Could you check a few things on this drawing? It's one solid part, dimensions in mm from its lowest x, y, z. A direction names the side the tool comes from. Give positions to 0.01 mm unless a question says otherwise; leave off trailing zeros. Write each loop counter-clockwise with the first axis right and the second up, starting at its lowest first coordinate (ties: lowest second). Pieces come first, ordered by that corner, then holes. Notation, with made-up numbers: M -40,45 L -8,45 A22 ccw -8,65 Z; hole C 47.25,8 d2. An arc over 180 degrees is marked long. Answer as CSV lines item,"result". Start each with the question number.
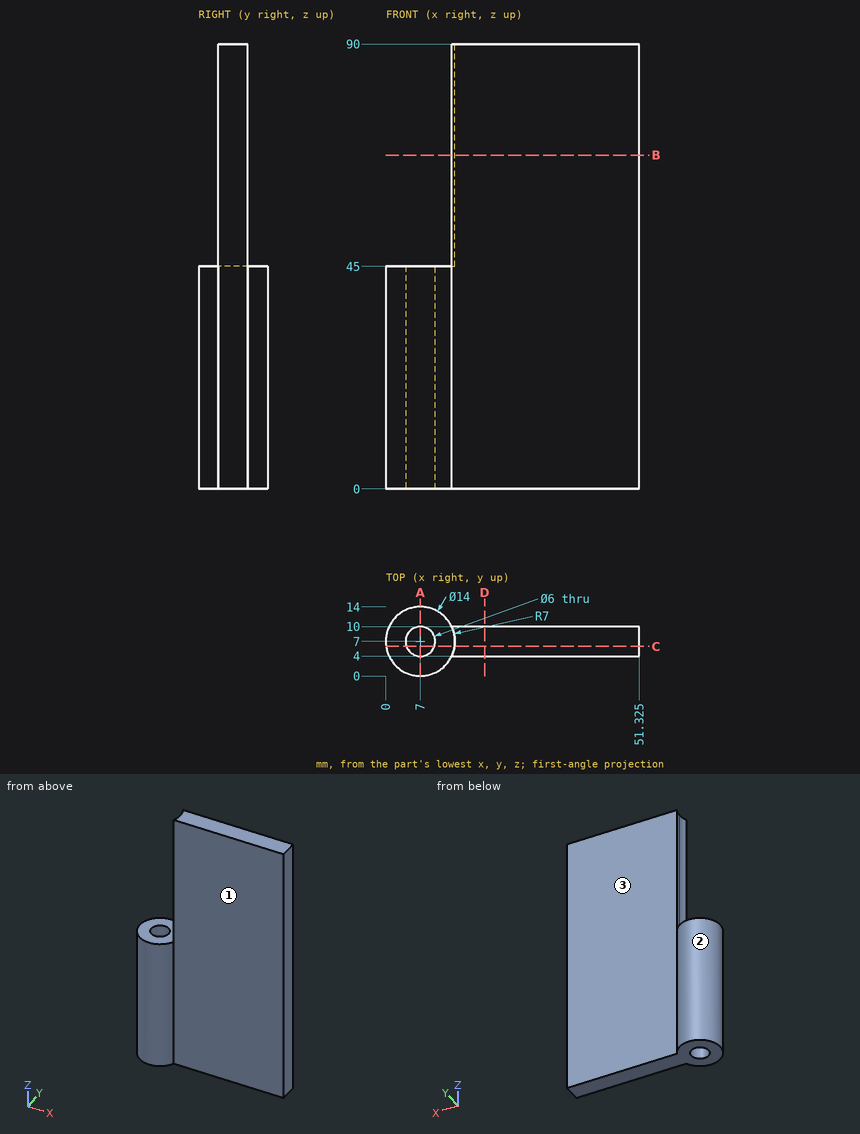
1) I want a section at A-A, the plane x = 7. Please give me the cut outline in (y, z).
2) I want a section at B-B, the plane z = 67.5. Please give me the cut outline in (x, y) (1 decimal).
3) I need wall thicknesses on L1, parallel to Y at x = 7, z = 15; L2, parallel to X at y = 7, z = 28 (1 decimal); L3, parallel to Z at x = 12, y = 11.5. Which ranges of each line are inside material? Lowest first, please. Write a range as from..to.
4) I want a section at D-D, the plane x = 20. Please give me the cut outline in (y, z), then the cut area to 3 significant figures.
5) I'm going to push flat-ended pins straight in: P1, Ø5, axis at y = 8.5, z = 20.5, coming from the -X side; P2, Ø6, axis at x = 10, y = 8.5, coming from the +Z side; P3, Ø1.5, axis at x = 20.5, z = 49, coming from the -Y side. Where does each tip first touch, or does it pass through?
6) I want a section at C-C, the plane y = 6. Please give me the cut outline in (x, z) (1 decimal).
7) On a 3-axis mill with a long thin cutter (end or side, diameter ignored), from which of +Z, -Z, +X, -X, +Y, -Y can I reach the whole of each face in a straight line? I mean the marked faces 1, 2 and 3. Say none if no direction works.
Values found:
1,outline,"M 0,0 L 4,0 L 4,45 L 0,45 Z; M 10,0 L 14,0 L 14,45 L 10,45 Z"
2,outline,"M 13.3,4 L 51.3,4 L 51.3,10 L 13.3,10 A7 cw 14,7 A7 cw Z"
3,L1,"y = 0..4, 10..14"
3,L2,"x = 0..4, 10..51.3"
3,L3,"z = 0..45"
4,outline,"M 4,0 L 10,0 L 10,90 L 4,90 Z"
4,area,"540 mm²"
5,P1,"stops at x = 0"
5,P2,"stops at z = 45"
5,P3,"stops at y = 4"
6,outline,"M 0.1,0 L 4.2,0 L 4.2,45 L 0.1,45 Z; M 9.8,0 L 51.3,0 L 51.3,90 L 13.9,90 L 13.9,45 L 9.8,45 Z"
7,face 1,"+Z, -Z, +X, -Y"
7,face 2,"+Z, -Z"
7,face 3,"+Z, -Z, +X, +Y"
